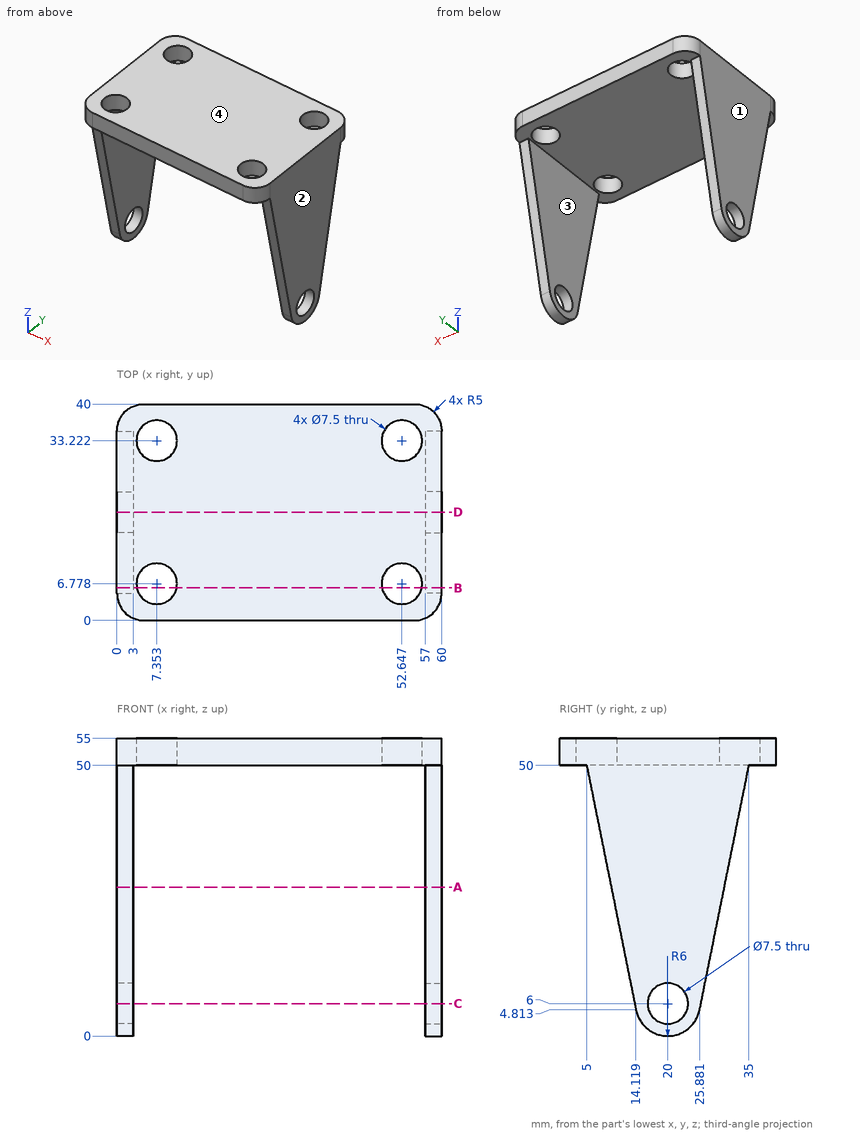
Could you check a few things on this drawing? It's one solid part, dimensions in mm from its lowest x, y, z. Round coordinates to 2 decimals unless told otherwise and drop trailing zeros. Write each loop counter-clockwise with the first axis right and the second up, starting at its lowest first coordinate (ties: lowest second). Pieces come first, ordered by that corner, then holes. Notation, with made-up numbers: (-3, 34.25) -> (45, 34.25) arc R19 cw to (45, 70.25) -> close; hole circle Ø4 at (56.5, 77.5). An arc over 180 degrees is marked (long way). One line per question, with ' | ' between items. Start each with the question number.
1) If we mould it in two halves opening along X, with no side actions, what happens to the marked faces 1, 2, 3 and 4? For each: released by +X, released by -X, zero draft, split by the parting line, or undercut.
2) Suppose I cut it at C-C on z = 6. Write out the boundary of the cut face in (x, y).
3) Suppose I cut it at A-A on z = 27.5. Write out the boundary of the cut face in (x, y).
4) I need wall thicknesses on line 1 (X direction, y = 27.5, z = 44.5); line 2 (Y direction, x = 8, z = 53) (1 decimal); line 3 (Z direction, x = 0.8, y = 20). Which ranges of each line are inside material? Lowest first, please. Write a range as [from, to].
5) Suppose I cut it at B-B on y = 6. Write out the boundary of the cut face in (x, z) (1 decimal), then the cut area to 3 significant figures.
6) Suppose I cut it at D-D on y = 20. Write out the boundary of the cut face in (x, z).
7) I'm going to push a flat-ended pin straight in: P1, Ø10, axis at x = 45, y = 20, coming from the -Z side. Where does the tip first touch, or does it pass through?
Return value:
1) face 1: released by -X | face 2: released by +X | face 3: undercut | face 4: zero draft
2) outline: (0, 13.88) -> (3, 13.88) -> (3, 16.25) -> (0, 16.25) -> close; (0, 23.75) -> (3, 23.75) -> (3, 26.12) -> (0, 26.12) -> close; (57, 13.88) -> (60, 13.88) -> (60, 16.25) -> (57, 16.25) -> close; (57, 23.75) -> (60, 23.75) -> (60, 26.12) -> (57, 26.12) -> close
3) outline: (0, 9.54) -> (3, 9.54) -> (3, 30.46) -> (0, 30.46) -> close; (57, 9.54) -> (60, 9.54) -> (60, 30.46) -> (57, 30.46) -> close
4) line 1: x = [0, 3], [57, 60] | line 2: y = [0, 3.1], [10.5, 29.5], [36.9, 40] | line 3: z = [0, 2.25], [9.75, 55]
5) outline: (0, 45) -> (3, 45) -> (3, 50) -> (3.7, 50) -> (3.7, 55) -> (0, 55) -> close; (11, 50) -> (49, 50) -> (49, 55) -> (11, 55) -> close; (56.3, 50) -> (57, 50) -> (57, 45) -> (60, 45) -> (60, 55) -> (56.3, 55) -> close | area: 256 mm2
6) outline: (0, 0) -> (3, 0) -> (3, 2.25) -> (0, 2.25) -> close; (0, 9.75) -> (3, 9.75) -> (3, 50) -> (57, 50) -> (57, 9.75) -> (60, 9.75) -> (60, 55) -> (0, 55) -> close; (57, 0) -> (60, 0) -> (60, 2.25) -> (57, 2.25) -> close
7) P1: stops at z = 50
